Part model, mm, in its own coordinate system. A direction names the side the tool comes from. Round coordinates to 2 decimals unless told otherwise and drop trailing zeros. Loops run counter-clockwise (first coordinate to the right, second up) from the corner with the lowest first, then second, coordinate; pieces in that order, holes last. Notation, with made-up numbers: (13, -38.75) -> (18, -38.75) arc R21 ccw to (18, -3.75) -> close; hole circle Ø4 at (46.25, 49.25). An arc over 180 degrees is marked (long way). Answer as a JSON object with one key per item and string values. Group by question number.
Autodesk Inventor part; units mm, degrees
ref_plane "YZ Plane" through (0, 0, 0) normal (1, 0, 0) x (0, 1, 0)
ref_plane "XZ Plane" through (0, 0, 0) normal (0, 1, 0) x (-1, 0, 0)
ref_plane "XY Plane" through (0, 0, 0) normal (0, 0, 1) x (1, 0, 0)
sketch "Sketch1" plane through (0, 0, 0) normal (0, 1, 0) x (-1, 0, 0)
  line L0 (0, 0) -> (431.8, 0)
  line L1 (431.8, 0) -> (431.8, -25.4)
  line L2 (431.8, -25.4) -> (0, -25.4)
  line L3 (0, -25.4) -> (0, 0)
  dimension "d0" = 431.8
  dimension "d1" = 25.4
extrude "Extrusion1" add sketch "Sketch1" along normal blind 3.429
sketch "Sketch2" plane through (0, 3.429, 0) normal (0, 1, 0) x (1, 0, 0)
  line L0 (0, 25.4) -> (-431.8, 25.4)
  line L1 (-44.45, 25.4) -> (-171.0436, 25.4)
  line L2 (-171.0436, 25.4) -> (-171.0436, 21.7932)
  line L3 (-171.0436, 21.7932) -> (-44.45, 21.7932)
  line L4 (-44.45, 21.7932) -> (-44.45, 25.4)
  line L5 (0, 0) -> (0, 25.4)
  point P0 (-44.45, 23.5966)
  dimension "d4" = 126.5936
  dimension "d5" = 3.6068
  dimension "d6" = 44.45
extrude "Extrusion2" add sketch "Sketch2" along normal blind 12.5984
sketch "Sketch3" plane through (0, 16.0274, 0) normal (0, 1, 0) x (1, 0, 0)
  line L0 (-431.8, 0) -> (0, 0)
  line L1 (0, 0) -> (0, 25.4)
  line L2 (0, 25.4) -> (-431.8, 25.4)
  line L3 (-431.8, 25.4) -> (-431.8, 0)
extrude "Extrusion3" add sketch "Sketch3" along normal blind 3.429
sketch "Sketch4" plane through (0, 19.4564, 0) normal (0, 1, 0) x (1, 0, 0)
  line L0 (0, 25.4) -> (-431.8, 25.4)
  line L1 (0, 0) -> (0, 25.4)
  line L2 (-431.8, 25.4) -> (-431.8, 0)
  point P0 (-12.7, 12.7)
  point P1 (-419.1, 12.7)
  point P2 (-317.5, 12.7)
  dimension "d11" = 12.7
  dimension "d12" = 12.7
  dimension "d13" = 12.7
  dimension "d14" = 12.7
  dimension "d15" = 12.7
  dimension "d24" = 114.3
hole "Hole1" at (-12.7, 19.4564, -12.7) at (-419.1, 19.4564, -12.7) at (-317.5, 19.4564, -12.7) direction (0, -1, 0) diameter 6.5024 end through all
sketch "Sketch5" plane through (0, 19.4564, 0) normal (0, 1, 0) x (1, 0, 0)
  point P0 (0, 0)
properties part number "ArmPart2.1"
Item 1: Band-saw the part on A-A, the plane x = -177. List the corners of the cut face in (y, z).
Item 2: Two-plate mould, pull along X, no slides. Class faces 3 (the face through (-15.924, 17.718, -13.123)), 4 (the face through (-219, 19.456, -13)): pulls with the +X half, pulls with the -X half, needs draft (parallel to the pull), parting line crosses it, or undercut.
Item 3: Drill centre lines: line 1 (X direction, y = 18.3, z = -12.7); line 2 (Y direction, x = -97, z = -9.75); line 3 (Z direction, x = -317.5, y = 18.6). Where is each one in solid material? Low to high.
Item 4: Band-saw the part on B-B, the plane y = 13. List the corners of the cut face in (x, z), plus the area to 3 significant figures.
Item 5: Which spindle directions (+Z, -Z, +X, -X, +Y, -Y) get a long thin tool onto all of the face, cutting with end or side? Do faces 1 (the face through (-320.724, 17.718, -13.123)), 2 (the face through (-109, 10, -21.793)). Say none if no direction does.
Item 6: Drop flat-ended pins along their axis: pin 1 Ø4 at (y, z) = (12.5, -23) entering from +X; pin 2 Ø4 at (x, y) = (-82.5, 6.5) entering from +Z; pin 3 Ø4 at (y, z) = (11.5, -23) entering from -X. Give the stop position or say it passes through.
Entries:
{
 "1": {"outline": "(0, -25.4) -> (3.43, -25.4) -> (3.43, 0) -> (0, 0) -> close; (16.03, -25.4) -> (19.46, -25.4) -> (19.46, 0) -> (16.03, 0) -> close"},
 "2": {"face 3": "undercut", "face 4": "needs draft"},
 "3": {"line 1": "-431.8 to -422.35, -415.85 to -320.75, -314.25 to -15.95, -9.45 to 0", "line 2": "0 to 3.43, 16.03 to 19.46", "line 3": "-25.4 to -15.95, -9.45 to 0"},
 "4": {"outline": "(-171.04, -25.4) -> (-44.45, -25.4) -> (-44.45, -21.79) -> (-171.04, -21.79) -> close", "area": "457 mm²"},
 "5": {"face 1": "+Y, -Y", "face 2": "+Z, +X, -X"},
 "6": {"pin 1": "x = -44.45", "pin 2": "z = -21.79", "pin 3": "x = -171.04"}
}
